Could you check a few things on this model? Use its own coordinates, in mm. A direction names the side the tool comes from. Round coordinates to 2 decimals unless told otherwise and drop trailing zeros. Write each loop counter-clockwise with the first axis right and the second up, starting at its lowest first coordinate (ties: lowest second). Pieces come first, ordered by that corner, then holes. Notation, with made-up numbers: (-10.75, 82.25) - (19.25, 82.25) arc R22 ccw to (19.25, 121.25) - close; hole circle Ø9 at (5.25, -33). An arc over 180 degrees is marked (long way). Put each result on its own line as item: value.
Autodesk Fusion 360 part; units mm, degrees
sketch "BasePlate" plane through (0, 0, 0) normal (0, 0, 1) x (1, 0, 0)
  line L0 (21.35, 9.5) -> (0, 9.5)
  line L1 (21.35, 9.5) -> (21.35, -9.5)
  line L2 (0, -9.5) -> (0, 9.5)
  line L3 (0, -9.5) -> (21.35, -9.5)
  line L4 (-2, 11.5) -> (23.35, 11.5)
  line L5 (23.35, 11.5) -> (23.35, -11.5)
  line L6 (23.35, -11.5) -> (-2, -11.5)
  line L7 (-2, -11.5) -> (-2, 11.5)
  line L8 (3, 6.5) -> (18.35, 6.5)
  line L9 (18.35, 6.5) -> (18.35, -6.5)
  line L10 (18.35, -6.5) -> (3, -6.5)
  line L11 (3, -6.5) -> (3, 6.5)
  dimension "d4" = 21.35
  dimension "d13" = 19
extrude "Extrude1" add sketch "BasePlate" along normal blind 2 contours L0 L1 L2 L3
extrude "Extrude2" add sketch "BasePlate" along normal blind 3 contours L4 L5 L6 L7
(1) I'm going to push a flat-ended pin straight in: pin 1 (12 mm diameter, centred on x = 15.5, y = -1, fed in from -Z). Where does the tip first touch, or does it pass through?
Values found:
pin 1: stops at z = 0
(2) Please list where these lines run through material, in increasing order: probe 1 along X at (y, z) = (-6, 0.65); probe 2 along Y at (x, z) = (18, 2.2); probe 3 along Y at (x, z) = (10, 0.8). Write a range as from..to.
Values found:
probe 1: x = -2..3, 18.35..23.35
probe 2: y = -11.5..-9.5, 9.5..11.5
probe 3: y = -11.5..-6.5, 6.5..11.5
(3) Imagine slicing it at C-C, the plane z = 2.55. List the corners of the cut face in (x, y) for me.
Values found:
outline: (-2, -11.5) - (23.35, -11.5) - (23.35, 11.5) - (-2, 11.5) - close; hole (0, -9.5) - (21.35, -9.5) - (21.35, 9.5) - (0, 9.5) - close
(4) For faces 1 (the face through (0, -0.1, 2.5)), 2 (the face through (18.35, 0, 1)), 3 (the face through (10, -10, 3)), which set-ups out of +Z, -Z, +X, -X, +Y, -Y let a thin tool reach every point of the face, with its end or its side?
Values found:
face 1: +Z
face 2: +Z, -Z
face 3: +Z, +X, -X, +Y, -Y
(5) Imagine slicing it at B-B, the plane y = 5.25. List the corners of the cut face in (x, z) for me.
Values found:
outline: (-2, 0) - (3, 0) - (3, 2) - (0, 2) - (0, 3) - (-2, 3) - close; (18.35, 0) - (23.35, 0) - (23.35, 3) - (21.35, 3) - (21.35, 2) - (18.35, 2) - close
(6) Imagine slicing it at A-A, the plane x = 16.5. List the corners of the cut face in (y, z) for me, then the cut area to 3 significant figures.
Values found:
outline: (-11.5, 0) - (-6.5, 0) - (-6.5, 2) - (-9.5, 2) - (-9.5, 3) - (-11.5, 3) - close; (6.5, 0) - (11.5, 0) - (11.5, 3) - (9.5, 3) - (9.5, 2) - (6.5, 2) - close
area: 24.0 mm^2
(7) If we mould it in two halves opening along X, with no side actions, what happens to faces 4 (the face through (-2, 0, 1)), 5 (the face through (23.35, 0, 1)), 6 (the face through (3, 0, 1))? For each: pulls with the +X half, pulls with the -X half, needs draft (parallel to the pull), parting line crosses it, or undercut.
Values found:
face 4: pulls with the -X half
face 5: pulls with the +X half
face 6: undercut
(8) Imagine slicing it at D-D, the plane y = -8.75. List the corners of the cut face in (x, z) for me, then the cut area to 3 significant figures.
Values found:
outline: (-2, 0) - (23.35, 0) - (23.35, 3) - (21.35, 3) - (21.35, 2) - (0, 2) - (0, 3) - (-2, 3) - close
area: 54.7 mm^2
